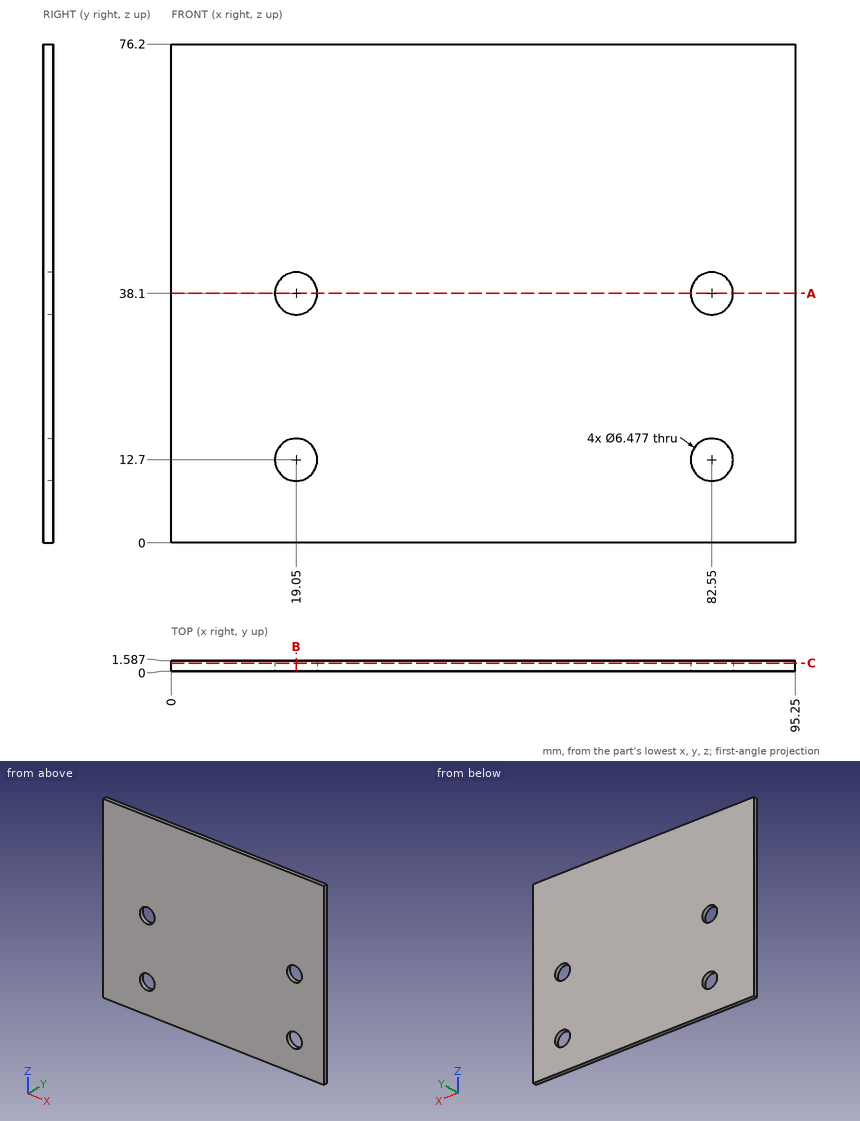
Print and shaded views of the part. All mm, measured from the part's lowest x, y and z. Give positions to 0.01 mm unless a question says otherwise; leave off trailing zeros. Loops run counter-clockwise (first coordinate to the right, second up) from the corner with the lowest first, then second, coordinate; pieces in that order, holes last.
1) Wall check: line 1 (X direction, y = 0.4, z = 12.7); line 2 (Z direction, x = 19.05, y = 0.65); line 3 (Z direction, x = 83.5, y = 0.55) (1 decimal). Give the ranges that are in metal, low to high.
2) Saw through at B-B (x = 19.05). Write the cut outline in (y, z).
3) Saw through at C-C (y = 1.25). Write the cut outline in (x, z), plus the area to 3 significant figures.
4) Saw through at A-A (z = 38.1). Write the cut outline in (x, y).
Answer block:
1. line 1: x = 0 to 15.81, 22.29 to 79.31, 85.79 to 95.25
1. line 2: z = 0 to 9.46, 15.94 to 34.86, 41.34 to 76.2
1. line 3: z = 0 to 9.6, 15.8 to 35, 41.2 to 76.2
2. outline: (0, 0) - (1.59, 0) - (1.59, 9.46) - (0, 9.46) - close; (0, 15.94) - (1.59, 15.94) - (1.59, 34.86) - (0, 34.86) - close; (0, 41.34) - (1.59, 41.34) - (1.59, 76.2) - (0, 76.2) - close
3. outline: (0, 0) - (95.25, 0) - (95.25, 76.2) - (0, 76.2) - close; hole circle Ø6.48 at (19.05, 12.7); hole circle Ø6.48 at (19.05, 38.1); hole circle Ø6.48 at (82.55, 12.7); hole circle Ø6.48 at (82.55, 38.1)
3. area: 7,130 mm2
4. outline: (0, 0) - (15.81, 0) - (15.81, 1.59) - (0, 1.59) - close; (22.29, 0) - (79.31, 0) - (79.31, 1.59) - (22.29, 1.59) - close; (85.79, 0) - (95.25, 0) - (95.25, 1.59) - (85.79, 1.59) - close
